Autodesk Inventor part; units mm, degrees
ref_plane "YZ Plane" through (0, 0, 0) normal (1, 0, 0) x (0, 1, 0)
ref_plane "XZ Plane" through (0, 0, 0) normal (0, 1, 0) x (-1, 0, 0)
ref_plane "XY Plane" through (0, 0, 0) normal (0, 0, 1) x (1, 0, 0)
sketch "Sketch1" plane through (0, 0, 0) normal (0, 0, 1) x (1, 0, 0)
  circle A0 centre (0, 0) radius 3.9
  circle A1 centre (0, 0) radius 3.75
  dimension "d0" = 7.5
extrude "Extrusion1" add sketch "Sketch1" along normal blind 2.55 contours A1
sketch "Sketch2" plane through (0, 0, 2.55) normal (0, 0, 1) x (1, 0, 0)
  arc A0 (-0.8298, -2.3052) -> (0.8298, -2.3052) centre (0, 0) ccw
  circle A1 centre (0, 0) radius 3.75
  circle A2 centre (0, 0) radius 3.75
  arc A3 (1.2702, -3.5283) -> (0.8298, -2.3052) centre (1.05, -2.9168) ccw
  arc A4 (-0.8298, -2.3052) -> (-1.2702, -3.5283) centre (-1.05, -2.9168) ccw
  line L0 (0, -2.45) -> (0, 0)
  dimension "d3" = 1.3
  dimension "d4" = 3.4
extrude "Extrusion2" add sketch "Sketch2" along normal blind 2 contours A0 A3 A1 A4 picked at (0, -3.3001)
sketch "Sketch3" plane through (0, 0, 2.55) normal (0, 0, 1) x (1, 0, 0)
  circle A0 centre (0, 0) radius 0.5
  dimension "d7" = 1
extrude "Extrusion3" cut sketch "Sketch3" against normal blind 2
properties part number "j024 output"
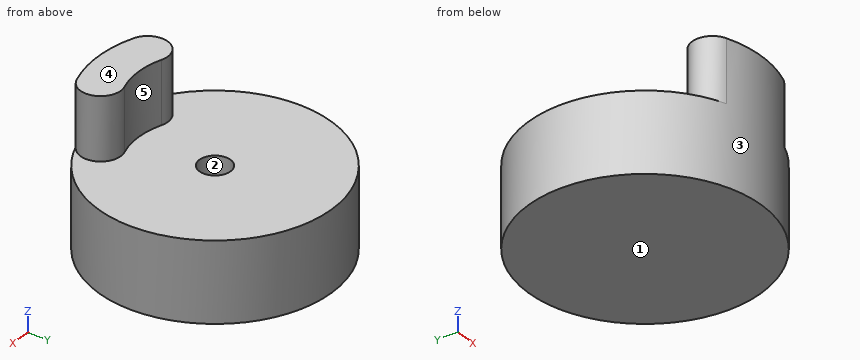
For this review, take the finished solid that the model builds, in its own axes (mm). Face numbers are marked on the shaded views. A direction names the side the tool comes from. Give positions to 0.01 mm unless a question says otherwise; leave off trailing zeros. Loops run counter-clockwise (first coordinate to the right, second up) from the corner with the lowest first, then second, coordinate; pieces in that order, holes last. Notation, with made-up numbers: (26, -33.75) - (30, -33.75) arc R26 ccw to (30, -9.75) - close; hole circle Ø7 at (53, 79.25). An arc over 180 degrees is marked (long way). Write each question's results on one line, items separated by ' | '.
(1) Take a section at B-B (z = 0.75). Give the boundary of the cut face in (x, y), then the cut area to 3 significant figures.
Conclusion:
outline: circle Ø7.5 at (0, 0); hole circle Ø1 at (0, 0) | area: 43.4 mm^2
(2) Take a section at D-D (y = -2.75). Give the boundary of the cut face in (x, z).
Conclusion:
outline: (-2.55, 0) - (2.55, 0) - (2.55, 2.55) - (1.68, 2.55) - (1.68, 4.55) - (-1.68, 4.55) - (-1.68, 2.55) - (-2.55, 2.55) - close
(3) Take a section at A-A (x = 0). Give the boundary of the cut face in (y, z), then the cut area to 3 significant figures.
Conclusion:
outline: (-3.75, 0) - (3.75, 0) - (3.75, 2.55) - (0.5, 2.55) - (0.5, 0.55) - (-0.5, 0.55) - (-0.5, 2.55) - (-2.45, 2.55) - (-2.45, 4.55) - (-3.75, 4.55) - close | area: 19.7 mm^2
(4) For line 1 along Y through (x, z) = (0, 1.9); line 2 along Z through (x, y) = (-0.5, -0.5); line 3 along Y through (x, z) = (1.25, 1.05), list the stretches that pass through material, from the lowest coordinate up.
Conclusion:
line 1: -3.75 to -0.5, 0.5 to 3.75 | line 2: 0 to 2.55 | line 3: -3.54 to 3.54
(5) Take a section at C-C (y = 0). Give the boundary of the cut face in (x, z).
Conclusion:
outline: (-3.75, 0) - (3.75, 0) - (3.75, 2.55) - (0.5, 2.55) - (0.5, 0.55) - (-0.5, 0.55) - (-0.5, 2.55) - (-3.75, 2.55) - close
(6) For the marked faces 4 and 5, list the 3-axis set-ups (+Z, -Z, +X, -X, +Y, -Y) from which the entire face can be reached by the end or side of a thin tool; tool diameter is ignored.
Conclusion:
face 4: +Z, +X, -X, +Y, -Y | face 5: +Z, +Y
(7) For pin 1 Ø2 at (x, y) = (3, -1) entering from +Z; pin 2 Ø3 at (x, y) = (-3, 1) entering from -Z, all flat-tipped, find the tip position at first contact; note any pin that passes through.
Conclusion:
pin 1: z = 2.55 | pin 2: z = 0
(8) Draft analysis for pull direction Y (two halves, no side actions). For the marked faces 1, 2 and 3, state which applies: +Y half, -Y half, draft (parallel to the pull), parting line (faces both ways), or undercut.
Conclusion:
face 1: draft | face 2: undercut | face 3: parting line
